Work out the finished part from the listing and answer in its coordinate system (mm). Round coordinates to 2 decimals unless told otherwise and drop trailing zeros. Write each loop counter-clockwise with the first axis right and the second up, starting at its lowest first coordinate (ties: lowest second). Pieces come first, ordered by that corner, then holes. Notation, with made-up numbers: (-37, -10) -> (3, -10) arc R10 cw to (3, -2) -> close; hole circle Ø8 at (71.5, -40). An arc over 180 degrees is marked (long way). One line per item, written item: value.
```python
from build123d import *

# Parameters (mm, degrees)
SKETCH1_R           = 8.89
BOSS_EXTRUDE1_DEPTH = 17.78
SKETCH3_R           = 1.5
CUT_EXTRUDE1_DEPTH  = 22.775963813
CIRPATTERN1_COUNT   = 2
CIRPATTERN1_ANGLE   = 90


with BuildPart() as part:
    # Sketch1 → Boss-Extrude1 (new body)
    with BuildSketch(Plane(origin=(0, 0, 0), x_dir=(1, 0, 0), z_dir=(0, 1, 0))):
        with Locations(Location((0, 0, 0), (0, 0, 270))):
            Circle(SKETCH1_R)
    extrude(amount=BOSS_EXTRUDE1_DEPTH)

    # Sketch2 → Cut-Revolve1 (revolve, cut)
    with BuildSketch(Plane.XY):
        with BuildLine():
            Line((0, 10.16), (0, 25.4))
            ThreePointArc((0, 25.4), (-7.62, 17.78), (0, 10.16))
        make_face()
    revolve(axis=Axis((0, 10.16, 0), (0, 1, 0)), mode=Mode.SUBTRACT)

    # Sketch3 → Cut-Extrude1 (cut, symmetric)
    with BuildSketch(Plane.XY):
        with Locations(Location((0, 3.81, 0), (0, 0, 90))):
            Circle(SKETCH3_R)
    cut_extrude1 = extrude(amount=CUT_EXTRUDE1_DEPTH, both=True, mode=Mode.SUBTRACT)

    # CirPattern1: Cut-Extrude1 ×2 about axis
    cirpattern1_axis = Axis((0, 0, 0), (0, 1, 0))
    for i in range(1, CIRPATTERN1_COUNT):
        add(cut_extrude1.rotate(cirpattern1_axis, i * CIRPATTERN1_ANGLE / (CIRPATTERN1_COUNT - 1)), mode=Mode.SUBTRACT)


solid = part.part
```
(1) Find section A-A on x = 0.25. Give the vertices of the cut face in (y, z), plus the area to 3 significant figures.
Reported:
outline: (0, -8.89) -> (2.33, -8.89) -> (2.33, -0.25) arc R1.5 cw to (2.33, 0.25) -> (2.33, 8.89) -> (0, 8.89) -> close; (5.29, -8.89) -> (17.78, -8.89) -> (17.78, -7.62) arc R7.62 cw to (17.78, 7.62) -> (17.78, 8.89) -> (5.29, 8.89) -> (5.29, 0.25) arc R1.5 cw to (5.29, -0.25) -> close
area: 172 mm2
(2) Find section C-C on z = 5.5. Give the vertices of the cut face in (x, y), plus the area to 3 significant figures.
Reported:
outline: (-6.98, 0) -> (6.98, 0) -> (6.98, 17.78) -> (5.27, 17.78) arc R5.27 cw to (-5.27, 17.78) -> (-6.98, 17.78) -> close; hole circle Ø3 at (0, 3.81)
area: 198 mm2
(3) Flat-ended cylindrical pins translate along their axes: pin 1 Ø4 at (x, y) = (0, 3.81) entering from -Z; pin 2 Ø6 at (y, z) = (9.5, -4) entering from -X; pin 3 Ø5 at (y, z) = (6.5, -4.5) entering from +X; pin 4 Ø4 at (x, y) = (-7, 10) entering from -Z. Find the tip coordinate at first contact, or state that the pin passes through.
Reported:
pin 1: stops at z = -8.89
pin 2: stops at x = -8.83
pin 3: stops at x = 8.66
pin 4: stops at z = -7.35
(4) For a pull along X with two mould halves and no side action, classify faces 1 (the face through (2.67, 8.77, 8.48)), 2 (the face through (-1.487, 3.615, 4.507)), 3 (the face through (-0.07, 2.31, -5.37)), 4 (the face through (0, 0, 0)) as pulls with the +X half, pulls with the -X half, needs draft (parallel to the pull), parting line crosses it, or undercut.
Reported:
face 1: parting line crosses it
face 2: undercut
face 3: undercut
face 4: needs draft
(5) Find section D-D on x = 6.5. Give the vertices of the cut face in (y, z).
Reported:
outline: (0, -6.06) -> (17.78, -6.06) -> (17.78, -3.98) arc R3.98 cw to (17.78, 3.98) -> (17.78, 6.06) -> (0, 6.06) -> close; hole circle Ø3 at (3.81, 0)
(6) Find section B-B on y = 3.81. Give the vertices of the cut face in (x, z), plus the area to 3 significant figures.
Reported:
outline: (-8.76, -1.5) arc R8.89 ccw to (-1.5, -8.76) -> (-1.5, -1.5) -> close; (-8.76, 1.5) -> (-1.5, 1.5) -> (-1.5, 8.76) arc R8.89 ccw to start; (1.5, -8.76) arc R8.89 ccw to (8.76, -1.5) -> (1.5, -1.5) -> close; (1.5, 1.5) -> (8.76, 1.5) arc R8.89 ccw to (1.5, 8.76) -> close
area: 151 mm2
(7) Consider probe 1 along Z at (x, y) = (4, 15.75); probe 2 along X at (y, z) = (3.81, 3.5); probe 3 along X at (y, z) = (3.81, -2.5). Determine where each line is inside the solid, lowest interval first.
Reported:
probe 1: z = -7.94 to -6.16, 6.16 to 7.94
probe 2: x = -8.17 to -1.5, 1.5 to 8.17
probe 3: x = -8.53 to -1.5, 1.5 to 8.53
